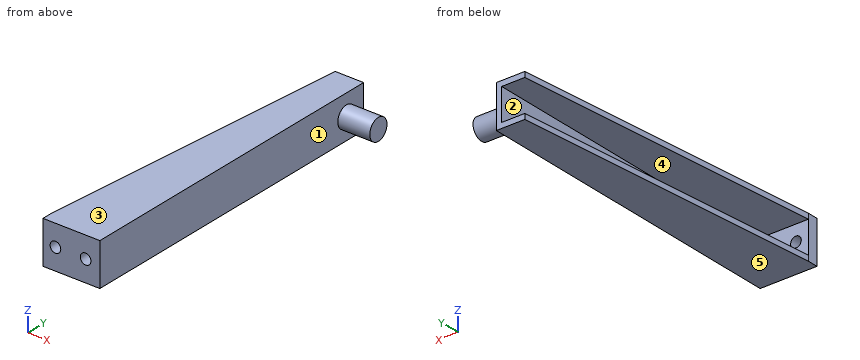
Autodesk Inventor part; units mm, degrees
ref_plane "YZ Plane" through (0, 0, 0) normal (1, 0, 0) x (0, 1, 0)
ref_plane "XZ Plane" through (0, 0, 0) normal (0, 1, 0) x (-1, 0, 0)
ref_plane "XY Plane" through (0, 0, 0) normal (0, 0, 1) x (1, 0, 0)
sketch "Boceto1" plane through (0, 0, 0) normal (0, 0, 1) x (1, 0, 0)
  line L0 (0, 0) -> (1.6, 0)
  line L1 (1.6, 0) -> (1.6, 0.3)
  line L2 (0, 0.3) -> (0, 0)
  line L3 (1.6, 0.3) -> (1.6, 8.287)
  line L4 (1.6, 8.287) -> (2.5, 8.287)
  line L5 (2.5, 8.287) -> (2.5, 8.887)
  line L6 (2.5, 8.887) -> (1.6, 8.887)
  line L7 (1.6, 8.887) -> (1.6, 9.187)
  line L8 (1.6, 9.187) -> (0.8, 9.187)
  line L9 (0.8, 9.187) -> (0, 0.3)
  line L10 (1.6, 8.887) -> (1.6, 8.287)
extrude "Extrusión1" add sketch "Boceto1" along normal blind 0.15 contours L2 L9 L8 L7 L10 L3 L1 L0
sketch "Boceto2" plane through (1.6, 0, 0) normal (1, 0, 0) x (0, 0, -1)
  line L0 (0, 0.3) -> (0, 9.187)
  line L1 (-1.2, 9.187) -> (-1.2, 0.3)
  line L2 (-1.2, 0.3) -> (0, 0.3)
  line L3 (-1.05, 0.3) -> (-1.05, 9.187)
  line L4 (-0.15, 0.3) -> (-0.15, 9.187)
  line L5 (-1.2, 0) -> (0, 0)
  line L6 (-1.2, 0) -> (-1.2, 0.3)
  line L7 (0, 0) -> (0, 0.3)
  line L8 (0, 9.187) -> (-1.2, 9.187)
  point P0 (0, 0)
extrude "Extrusión2" add sketch "Boceto2" against normal blind 0.15 contours L7 L5 L6 L2 | L2 L3 L8 L4 | L2 L1 L8 L3
sketch "Boceto3" plane through (1.6, 0, 1.2) normal (0, 0, 1) x (1, 0, 0)
  line L0 (-1.6, 0) -> (0, 0)
  line L1 (0, 0) -> (0, 0.3)
  line L2 (-1.6, 0.3) -> (-1.6, 0)
  line L3 (0, 0.3) -> (0, 8.287)
  line L4 (0, 8.287) -> (0.9, 8.287)
  line L5 (0.9, 8.287) -> (0.9, 8.887)
  line L6 (0.9, 8.887) -> (0, 8.887)
  line L7 (0, 8.887) -> (0, 9.187)
  line L8 (0, 9.187) -> (-0.8, 9.187)
  line L9 (-0.8, 9.187) -> (-1.6, 0.3)
  line L10 (0, 8.887) -> (0, 8.287)
  line L11 (0, 0) -> (-0.15, 0)
  point P0 (-1.6, 0)
extrude "Extrusión3" add sketch "Boceto3" against normal blind 0.15 contours L2 L9 L8 L7 L10 L3 L1 L0
sketch "Boceto4" plane through (1.45, 0, 0) normal (-1, 0, 0) x (0, 0, 1)
  line L0 (1.2, 0.3) -> (1.2, 9.187)
  line L1 (0, 9.187) -> (0, 0.3)
  line L2 (0, 0.3) -> (1.2, 0.3)
  line L3 (0.15, 0.3) -> (0.15, 9.187)
  line L4 (1.05, 0.3) -> (1.05, 9.187)
  line L5 (0, 0) -> (1.2, 0)
  line L6 (0, 0) -> (0, 0.3)
  line L7 (1.2, 0) -> (1.2, 0.3)
  line L8 (1.2, 9.187) -> (0, 9.187)
  point P0 (0, 0)
extrude "Extrusión4" add sketch "Boceto4" along normal blind 1.45 contours L7 L5 L6 L2
sketch "Boceto5" plane through (1.45, 0.3, 1.05) normal (0, 1, 0) x (1, 0, 0)
  line L0 (-1.45, 1.05) -> (0.15, 1.05)
  line L1 (0.15, 1.05) -> (0.15, -0.15)
  line L2 (0.15, -0.15) -> (-1.45, -0.15)
  line L3 (-1.45, -0.15) -> (-1.45, 1.05)
  circle A0 centre (-1.1, 0.45) radius 0.15
  circle A1 centre (-0.25, 0.45) radius 0.15
  line L4 (0.15, 0.15) -> (1.05, 0.15)
  line L5 (1.05, 0.15) -> (1.05, 0.75)
  line L6 (1.05, 0.75) -> (0.15, 0.75)
  line L7 (0, 1.05) -> (0, -0.15)
  line L8 (0.15, 1.05) -> (0.15, -0.15)
  point P0 (-1.45, 1.05)
extrude "Extrusión5" cut sketch "Boceto5" against normal blind 1.45 contours A0 | A1
sketch "Boceto6" plane through (1.6, 0, 0) normal (1, 0, 0) x (0, 0, -1)
  line L0 (0, 0) -> (-1.2, 0)
  line L1 (0, 0) -> (0, 9.187)
  line L2 (0, 9.187) -> (-1.2, 9.187)
  line L3 (-1.2, 9.187) -> (-1.2, 0)
  line L4 (0, 0.3) -> (0, 9.187)
  line L5 (-1.2, 9.187) -> (-1.2, 0.3)
  line L6 (-1.2, 0) -> (0, 0)
  line L7 (-1.2, 0) -> (-1.2, 0.3)
  line L8 (0, 0) -> (0, 0.3)
  line L9 (0, 9.187) -> (-1.2, 9.187)
  circle A0 centre (-0.6, 8.587) radius 0.3
extrude "Extrusión6" add sketch "Boceto6" along normal blind 0.9 contours A0
properties part number "soporteAgarre"
The model under review builds one solid part; all positions refer to its coordinate system, in mm. Face numbers are marked on the shaded views. A direction names the side the tool comes from. Give positions to 0.01 mm unless a question says otherwise; leave off trailing zeros. Loops run counter-clockwise (first coordinate to the right, second up) from the corner with the lowest first, then second, coordinate; pieces in that order, holes last. Notation, with made-up numbers: (86.5, -36.5) -> (115.5, -36.5) arc R16 cw to (115.5, -26.5) -> close; hole circle Ø6 at (29, 81). An arc over 180 degrees is marked (long way). Answer as a JSON object with one key per item and string values. Group by question number.
Q1. Take a section at C-C (y = 6.25). Write out the cut boundary in (x, z), plus the area to 3 significant figures.
Q2. Insertion check: pin 1 (0.5 mm diameter, centred on y = 6.5, z = 0.5, fed in from -X). The pin has a flat end and moves straight along its axis. Give the tip position at first contact, or say it passes through.
Q3. Tool access review of the marked faces 4 and 5: name each direction out of +Z, -Z, +X, -X, +Y, -Y from which nothing blocks a thin tool from reaching the whole face with its end or side.
Q4. Draft analysis for pull direction Z (two halves, no side actions). For the marked faces 1, 2 and 3, state which applies: pulls with the +Z half, pulls with the -Z half, needs draft (parallel to the pull), parting line crosses it, or undercut.
Q5. Wall thickness on line 1 along X through (y, z) = (0.2, 0.6); line 2 along Z through (x, y) = (1.2, 0.15); line 3 along X through (y, z) = (1, 0.7): over which ranges is each line inside the solid? List them lowest first.
Q6. Take a section at B-B (x = 1.2). Write out the cut boundary in (y, z), plus the area to 3 significant figures.
Q7. Take a section at A-A (z = 0.6). Write out the cut boundary in (x, y).
Q8. Take a section at D-D (x = 0.3). Write out the cut boundary in (y, z), plus the area to 3 significant figures.
Answer below:
{
 "1": {"outline": "(0.54, 0) -> (1.6, 0) -> (1.6, 1.2) -> (0.54, 1.2) -> (0.54, 1.05) -> (1.45, 1.05) -> (1.45, 0.15) -> (0.54, 0.15) -> close", "area": "0.454 mm2"},
 "2": {"pin 1": "stops at x = 1.45"},
 "3": {"face 4": "-X, +Y", "face 5": "-Z, +X, -X, +Y, -Y"},
 "4": {"face 1": "needs draft", "face 2": "undercut", "face 3": "pulls with the +Z half"},
 "5": {"line 1": "x = 0 to 0.2, 0.5 to 1.05, 1.35 to 1.6", "line 2": "z = 0 to 0.45, 0.75 to 1.2", "line 3": "x = 1.45 to 1.6"},
 "6": {"outline": "(0, 0) -> (9.19, 0) -> (9.19, 0.15) -> (0.3, 0.15) -> (0.3, 0.45) -> (0, 0.45) -> close; (0, 0.75) -> (0.3, 0.75) -> (0.3, 1.05) -> (9.19, 1.05) -> (9.19, 1.2) -> (0, 1.2) -> close", "area": "2.94 mm2"},
 "7": {"outline": "(0, 0) -> (0.2, 0) -> (0.2, 0.3) -> (0, 0.3) -> close; (0.5, 0) -> (1.05, 0) -> (1.05, 0.3) -> (0.5, 0.3) -> close; (1.35, 0) -> (1.6, 0) -> (1.6, 8.29) -> (2.5, 8.29) -> (2.5, 8.89) -> (1.6, 8.89) -> (1.6, 9.19) -> (1.45, 9.19) -> (1.45, 0.3) -> (1.35, 0.3) -> close"},
 "8": {"outline": "(0, 0) -> (3.63, 0) -> (3.63, 0.15) -> (0.3, 0.15) -> (0.3, 0.46) -> (0, 0.46) -> close; (0, 0.74) -> (0.3, 0.74) -> (0.3, 1.05) -> (3.63, 1.05) -> (3.63, 1.2) -> (0, 1.2) -> close", "area": "1.27 mm2"}
}
